```python
from build123d import *

# Parameters (mm, degrees)
SKETCH1_R           = 7
SKETCH1_R_2         = 2.75
SKETCH1_R_3         = 3.659852489
BOSS_EXTRUDE1_DEPTH = 7
SKETCH2_R           = 8
SKETCH2_R_2         = 6
BOSS_EXTRUDE2_DEPTH = 17
FILLET1_R           = 3
FILLET2_R           = 3
SKETCH3_R           = 1


with BuildPart() as part:
    # Sketch1 → Boss-Extrude1 (new body)
    with BuildSketch(Plane(origin=(0, 0, 0), x_dir=(1, 0, 0), z_dir=(0, 1, 0))):
        with BuildLine():
            ThreePointArc((-15.634333704, 6.748663161), (-22.25, 0), (-15.634333704, -6.748663161))
            ThreePointArc((-15.634333704, -6.748663161), (-12.054001616, -7.488359295), (-8.978814065, -9.465516285))
            ThreePointArc((-8.978814065, -9.465516285), (-0.448762307, -12.99442036), (8.273320847, -9.971141939))
            ThreePointArc((8.273320847, -9.971141939), (11.493139678, -8.165901558), (15.148520579, -7.651784261))
            ThreePointArc((15.148520579, -7.651784261), (23.159852489, 0), (15.148520579, 7.651784261))
            ThreePointArc((15.148520579, 7.651784261), (11.493139678, 8.165901558), (8.273320847, 9.971141939))
            ThreePointArc((8.273320847, 9.971141939), (-0.448762307, 12.99442036), (-8.978814065, 9.465516285))
            ThreePointArc((-8.978814065, 9.465516285), (-12.054001616, 7.488359295), (-15.634333704, 6.748663161))
        make_face()
        with Locations(Location((0, 0, 0), (0, 0, 270))):
            Circle(SKETCH1_R, mode=Mode.SUBTRACT)
        with Locations(Location((-15.5, 0, 0), (0, 0, 270))):
            Circle(SKETCH1_R_2, mode=Mode.SUBTRACT)
        with Locations(Location((15.5, 0, 0), (0, 0, 270))):
            Circle(SKETCH1_R_3, mode=Mode.SUBTRACT)
    extrude(amount=BOSS_EXTRUDE1_DEPTH)

    # Sketch2 → Boss-Extrude2 (add)
    with BuildSketch(Plane(origin=(0, 7, 0), x_dir=(1, 0, 0), z_dir=(0, 1, 0))):
        with Locations(Location((0, 0, 0), (0, 0, 270))):
            Circle(SKETCH2_R)
        with Locations(Location((0, 0, 0), (0, 0, 270))):
            Circle(SKETCH2_R_2, mode=Mode.SUBTRACT)
    extrude(amount=BOSS_EXTRUDE2_DEPTH)

    # Fillet1
    # the kernel refuses this fillet: 3 mm, written as the material it adds along each edge
    with BuildSketch(Plane(origin=(0, 7, 0), x_dir=(0, 0, 1), z_dir=(-1, 0, 0))) as fillet1_piece_1:
        with BuildLine():
            CenterArc((4, -2.236067977), FILLET1_R, 0, 48.189685104)
            Line((6, 0), (6.04, 0.04472136))
            ThreePointArc((6.04, 0.04472136), (6.5, 0.06), (7, 0.06))
            Line((7, 0.06), (7.06, 0))
            Line((7.06, 0), (7.06, -2.236067977))
            Line((7.06, -2.236067977), (7, -2.236067977))
        make_face()
    revolve(axis=Axis((0, 7, 0), (0, 1, 0)))
    with BuildSketch(Plane(origin=(0, 7, 0), x_dir=(0, 0, 1), z_dir=(-1, 0, 0))) as fillet1_piece_2:
        with BuildLine():
            CenterArc((8 + FILLET1_R, FILLET1_R), FILLET1_R, 180, 90)
            Line((8, FILLET1_R), (8 - FILLET1_R * 0.02, FILLET1_R))
            Line((8 - FILLET1_R * 0.02, FILLET1_R), (8 - FILLET1_R * 0.02, -FILLET1_R * 0.02))
            Line((8 - FILLET1_R * 0.02, -FILLET1_R * 0.02), (8 + FILLET1_R, -FILLET1_R * 0.02))
            Line((8 + FILLET1_R, -FILLET1_R * 0.02), (8 + FILLET1_R, 0))
        make_face()
    revolve(axis=Axis((0, 7, 0), (0, 1, 0)))

    # Fillet2
    fillet2_edges = [part.edges().sort_by_distance(p)[0] for p in [
        (0, 7, -6),
    ]]
    fillet(fillet2_edges, radius=FILLET2_R)


with BuildPart() as body_2:
    # Sketch3 → Revolve1 (revolve)
    with BuildSketch(Plane(origin=(0, 0, 0), x_dir=(0, 0, -1), z_dir=(1, 0, 0))):
        with Locations((8.5, 19.608844607)):
            Circle(SKETCH3_R)
    revolve(axis=Axis((0, 0, 0), (0, 1, 0)))


with BuildPart() as part_1:
    add(part.part)

    # Intersect1: read off the stored shape, not the designer's step
    # Intersect1: cut body 2
    add(body_2.part, mode=Mode.SUBTRACT)


solid = part_1.part
```
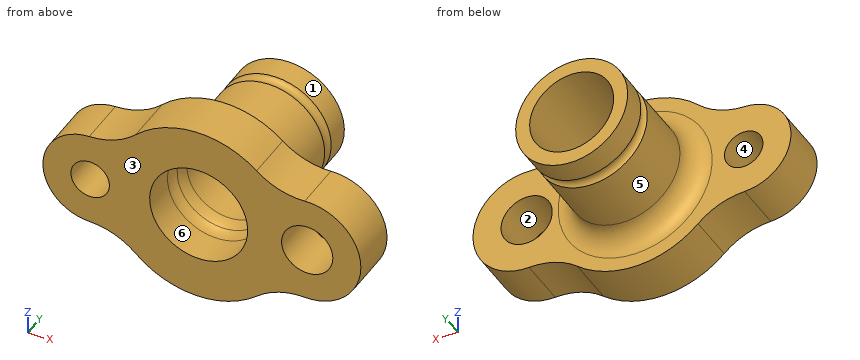
The listing builds one solid part. Answer for the finished solid, in the listing's coordinates (mm). Face numbers are marked on the shaded views. A direction names the side the tool comes from. Coordinates: 2 decimals unless noted, no trailing zeros. Write each loop counter-clockwise with the first axis right and the second up, starting at its lowest first coordinate (ties: lowest second). Pieces come first, ordered by that corner, then holes. Notation, with made-up numbers: (-37, -4.5) - (11, -4.5) arc R5 ccw to (11, -0.5) - close; hole circle Ø6 at (4, 14.5). An arc over 180 degrees is marked (long way). Return JSON: item names as keys, results as strings. Group by question number.
Q1. Flat-ended cylindrical pins translate along their axes: pin 1 Ø10 at (y, z) = (17.5, 4) entering from -X; pin 2 Ø6 at (x, y) = (11.5, 17.5) entering from +Z; pin 3 Ø2 at (x, y) = (-2, 3) entering from +Z; pin 4 Ø1.5 at (y, z) = (16, -7) entering from +X. Find the tip coordinate at first contact, or state that the pin passes through.
Q2. Find the intervals of material crossed by line 1 along X through (y, z) = (3.1, 0); line 2 along X through (y, z) = (16.5, 0); line 3 along X through (y, z) = (4.25, -2.25), in increasing order. Write a range as [from, to].
Q3. Which of the six approach directions +Z, -Z, +X, -X, +Y, -Y give full straight-line access (tool end or side, diameter ignored) to the marked faces 4, 5 and 6?
Q4. For a pull along Z with two mould halves and no side action, classify the marked faces 1, 2 and 3 as +Z half, -Z half, draft (parallel to the pull), parting line (faces both ways), or undercut.
Q5. The part is cut by section D-D on y = 21.25. Write down the section's boundary in (x, z), and give its area (3 significant figures).
Q6. The part is cut by section C-C on z = 0. State how many separate pieces and enclosed holes the cut face has, and give its area (3 significant figures).
Q7. The part is cut by section A-A on x = 12.5. Write down the section's boundary in (y, z).
Q8. The part is cut by section B-B on y = 2.5. Write down the section's boundary in (x, z).
Evaluation:
{
 "1": {"pin 1": "stops at x = -8", "pin 2": "passes through", "pin 3": "stops at z = 12.97", "pin 4": "stops at x = 4.99"},
 "2": {"line 1": "x = [-22.25, -18.25], [-12.75, -7], [7, 11.84], [19.16, 23.16]", "line 2": "x = [-8, -6], [6, 8]", "line 3": "x = [-21.86, -17.08], [-13.92, -6.63], [6.63, 12.61], [18.39, 22.82]"},
 "3": {"face 4": "+Y, -Y", "face 5": "+Y", "face 6": "-Y"},
 "4": {"face 1": "parting line", "face 2": "undercut", "face 3": "draft"},
 "5": {"outline": "circle Ø16 at (0, 0); hole circle Ø12 at (0, 0)", "area": "88.0 mm2"},
 "6": {"separate pieces": "4", "enclosed holes": "0", "area": "202 mm2"},
 "7": {"outline": "(0, -7.88) - (7, -7.88) - (7, -2.1) - (0, -2.1) - close; (0, 2.1) - (7, 2.1) - (7, 7.88) - (0, 7.88) - close"},
 "8": {"outline": "(-15.63, -6.75) arc R10 cw to (-8.98, -9.47) arc R13 ccw to (8.27, -9.97) arc R10 cw to (15.15, -7.65) arc R7.66 ccw (long way) to (15.15, 7.65) arc R10 cw to (8.27, 9.97) arc R13 ccw to (-8.98, 9.47) arc R10 cw to (-15.63, 6.75) arc R6.75 ccw to start; hole circle Ø5.5 at (-15.5, 0); hole circle Ø14 at (0, 0); hole circle Ø7.32 at (15.5, 0)"}
}
